```python
from build123d import *

# Parameters (mm, degrees)
BOSS_EXTRUDE1_DEPTH = 42
SKETCH3_R           = 10
BOSS_EXTRUDE2_DEPTH = 7
SKETCH4_R           = 6
CUT_EXTRUDE1_DEPTH  = 69.942004613
FILLET1_R           = 4


with BuildPart() as part:
    # Sketch1 → Boss-Extrude1 (new body)
    with BuildSketch(Plane.XY):
        Polygon((0, 0), (0, -6), (14, -6), (14, 14), (-35, 14), (-35, 0), align=None)
    extrude(amount=BOSS_EXTRUDE1_DEPTH)

    # Sketch3 → Boss-Extrude2 (add)
    with BuildSketch(Plane.ZY.offset(28)):
        with BuildLine():
            Line((0, 14), (42, 14))
            Line((42, 14), (42, 35))
            ThreePointArc((42, 35), (21, 56), (0, 35))
            Line((0, 35), (0, 14))
        make_face()
        with Locations((21, 35)):
            Circle(SKETCH3_R, mode=Mode.SUBTRACT)
    extrude(amount=BOSS_EXTRUDE2_DEPTH)

    # Sketch4 → Cut-Extrude1 (cut, through all)
    with BuildSketch(Plane(origin=(0, 14, 0), x_dir=(1, 0, 0), z_dir=(0, 1, 0))):
        with Locations(Location((-10, -21, 0), (0, 0, 180))):
            Circle(SKETCH4_R)
    extrude(amount=-CUT_EXTRUDE1_DEPTH, mode=Mode.SUBTRACT)

    # Fillet1
    fillet1_edges = [part.edges().sort_by_distance(p)[0] for p in [
        (14, 14, 21),
        (-28, 14, 21),
    ]]
    fillet(fillet1_edges, radius=FILLET1_R)

    # Mirror2: part across plane


with BuildPart() as part_1:
    add(part.part)
    add(part.part.mirror(Plane(origin=(-35, 14, 42), x_dir=(0, 0, 1), z_dir=(1, 0, 0))))


solid = part_1.part
```
Could you check a few things on this model? Use its own coordinates, in mm. A direction names the side the tool comes from. Give positions to 0.01 mm unless a question says otherwise; leave off trailing zeros. Loops run counter-clockwise (first coordinate to the right, second up) from the corner with the lowest first, then second, coordinate; pieces in that order, holes last. Notation, with made-up numbers: (77.25, 83) - (114.25, 83) arc R16 ccw to (114.25, 90) - close; hole circle Ø8 at (81.25, 17). An arc over 180 degrees is marked (long way). Answer in a Markdown table with one row per item. Add a question column.
Q1. If we section it at A-A (x = -10): List the corners of the cut face in (y, z) for me, plus the area to 3 significant figures.
Q2. Which directions (+Z, -Z, +X, -X, +Y, -Y) give clear straight access to the entire face, cutting with the end or side of a thin tool? Please do faces 1 (the face through (-42, 46, 21)), 2 (the face through (-3, 14, 21)), 3 (the face through (-35, 0, 21)), 4 (the face through (-35.098, 26.128, 25.614)), 5 (the face through (-77, -6, 21)).
Q3. If we section it at D-D (z = 33.5): List the corners of the cut face in (x, y) for me.
Q4. If we section it at B-B (z = 21): List the corners of the cut face in (x, y) for me, plus the area to 3 significant figures.
Q5. If we section it at C-C (y = 44): List the corners of the cut face in (x, z) for me.
Q6. Please list where these lines run through material, in increasing order: L1, parallel to Z at x = -60, y = 5; L2, parallel to X at y = -3, z = 25; L3, parallel to Y at x = -68.5, z = 37. Write a range as from..to.
Q7. For pin 1 (4 mm diameter, centred on x = -7, z = 26, fed in from +Y); pin 2 (1 mm diameter, centred on x = -43.5, z = 25.5, fed in from +Y); pin 3 (7 mm diameter, centred on x = -10, z = 21, fed in from +Y); pin 4 (5 mm diameter, centred on x = -50, z = 14, fed in from -Y), each with a flat end and sliding along its axis, tell me the tip position at first contact or that it passes through.
Q8. We'd pull the mould along Z, two halves only. Please class faces 6 (the face through (-66, 7, 21)), 7 (the face through (-36, 6, 0)), 8 (the face through (7, -6, 21)): +Z half, -Z half, draft (parallel to the pull), parting line (faces both ways), or undercut.
The answers:
| question | item | result |
|---|---|---|
| 1 | outline | (0, 0) - (14, 0) - (14, 15) - (0, 15) - close; (0, 27) - (14, 27) - (14, 42) - (0, 42) - close |
| 1 | area | 420 mm^2 |
| 2 | face 1 | +Z, -Z, -X, +Y |
| 2 | face 2 | +Z, -Z, +X, +Y |
| 2 | face 3 | +Z, -Z, -Y |
| 2 | face 4 | +X, -X |
| 2 | face 5 | +Z, -Z, +X, -X, -Y |
| 3 | outline | (-84, -6) - (-70, -6) - (-70, 0) - (0, 0) - (0, -6) - (14, -6) - (14, 10) arc R4 ccw to (10, 14) - (-24, 14) arc R4 cw to (-28, 18) - (-28, 51.87) - (-42, 51.87) - (-42, 18) arc R4 cw to (-46, 14) - (-80, 14) arc R4 ccw to (-84, 10) - close |
| 4 | outline | (-84, -6) - (-70, -6) - (-70, 0) - (-66, 0) - (-66, 14) - (-80, 14) arc R4 ccw to (-84, 10) - close; (-54, 0) - (-16, 0) - (-16, 14) - (-24, 14) arc R4 cw to (-28, 18) - (-28, 25) - (-42, 25) - (-42, 18) arc R4 cw to (-46, 14) - (-54, 14) - close; (-42, 45) - (-28, 45) - (-28, 56) - (-42, 56) - close; (-4, 0) - (0, 0) - (0, -6) - (14, -6) - (14, 10) arc R4 ccw to (10, 14) - (-4, 14) - close |
| 4 | area | 1,510 mm^2 |
| 5 | outline | (-42, 2.03) - (-28, 2.03) - (-28, 16.64) - (-42, 16.64) - close; (-42, 25.36) - (-28, 25.36) - (-28, 39.97) - (-42, 39.97) - close |
| 6 | L1 | z = 0..15, 27..42 |
| 6 | L2 | x = -84..-70, 0..14 |
| 6 | L3 | y = 0..14 |
| 7 | pin 1 | stops at y = 14 |
| 7 | pin 2 | stops at y = 15.35 |
| 7 | pin 3 | passes through |
| 7 | pin 4 | stops at y = 0 |
| 8 | face 6 | undercut |
| 8 | face 7 | -Z half |
| 8 | face 8 | draft |
